For this review, take the finished solid that the model builds, in its own axes (mm). A direction names the side the tool comes from. Give positions to 0.01 mm unless a question says otherwise; leave off trailing zeros. Order: outer loops, then holes, each group sorted by start corner. A loop starts at its lowest first (then second) coordinate and runs counter-clockwise, first axis right, second up.
Item 1: For probe 1 along Y at (x, z) = (11.5, 2); probe 2 along Z at (x, y) = (48.5, 11); probe 3 along Y at (x, z) = (38.5, 4.5), list the stretches that pass through material, from the lowest coordinate up.
Item 2: Consider section C-C (y = -79). Give the boundary of the cut face in (x, z).
Item 3: Consider section B-B (x = 6). Give the boundary of the cut face in (y, z), plus the area to 3 significant figures.
Item 4: The part is to be moulded in two halves that separate along X. For faces 1 (the flat face through (-86.994, -51.168, 5.465)), 2 (the flat face through (-1, 1, 20)), 3 (the flat face through (-1, 102, 3)), 4 (the flat face through (-60.854, -102.443, -3.055)), say which applies: released by +X, released by -X, zero draft, split by the parting line, or undercut.
Item 5: Machinability: for faces 5 (the flat face through (60.854, 102.443, -3.055)), 6 (the flat face through (-0.79, -91.21, 13.47)), 7 (the flat face through (-1, 100.923, 5)), 8 (the flat face through (87.81, -49.755, 5.465)), which of the approach directions +Z, -Z, +X, -X, +Y, -Y give a long, thin tool a straight path to every point of the face, cutting with its end or side? Answer none if there is none.
Item 6: Consider section A-A (z = 15). Give the boundary of the cut face in (x, y).
Item 7: For P1, Ø1.5, axis at x = -19.5, z = 2, coming from the -Y side; P2, Ø3, axis at x = -25.5, z = 14, coming from the +Y side; P3, Ø2.5, axis at x = -120, y = -4.5, coming from the +Z side, all flat-tipped, find the tip position at first contact; note any pin that passes through.
Autodesk Inventor part; units mm, degrees
ref_plane "YZ Plane" through (0, 0, 0) normal (1, 0, 0) x (0, 1, 0)
ref_plane "XZ Plane" through (0, 0, 0) normal (0, 1, 0) x (-1, 0, 0)
ref_plane "XY Plane" through (0, 0, 0) normal (0, 0, 1) x (1, 0, 0)
ref_plane "Plano de trabajo1" through (0, 0, 0) normal (0, 0, 1) x (1, 0, 0)
sketch "Boceto1" plane through (0, 0, 0) normal (0, 0, 1) x (1, 0, 0)
  line L0 (58.8453, 101.923) -> (-58.8453, 101.923)
  line L1 (-58.8453, 101.923) -> (-117.6906, 0)
  line L2 (-117.6906, 0) -> (-58.8453, -101.923)
  line L3 (-58.8453, -101.923) -> (58.8453, -101.923)
  line L4 (58.8453, -101.923) -> (117.6906, 0)
  line L5 (117.6906, 0) -> (58.8453, 101.923)
  line L6 (-60, 103.923) -> (-120, 0)
  line L7 (-120, 0) -> (-60, -103.923)
  line L8 (-60, -103.923) -> (60, -103.923)
  line L9 (60, -103.923) -> (120, 0)
  line L10 (120, 0) -> (60, 103.923)
  line L11 (60, 103.923) -> (-60, 103.923)
  line L12 (58.8453, 101.923) -> (117.6906, 0)
  line L13 (117.6906, 0) -> (58.8453, -101.923)
  line L14 (58.8453, -101.923) -> (-58.8453, -101.923)
  line L15 (-58.8453, -101.923) -> (-117.6906, 0)
  line L16 (-117.6906, 0) -> (-58.8453, 101.923)
  line L17 (-58.8453, 101.923) -> (58.8453, 101.923)
  point P0 (0, 0)
extrude "Extrusión1" add sketch "Boceto1" along normal blind 3 contours L5 L4 L3 L2 L1 L0 | L11 L10 L9 L8 L7 L6
sketch "Boceto2" plane through (0, 0, 3) normal (0, 0, 1) x (1, 0, 0)
  line L0 (-120, 0) -> (-60, -103.923)
  line L1 (-60, -103.923) -> (60, -103.923)
  line L2 (60, -103.923) -> (120, 0)
  line L3 (120, 0) -> (60, 103.923)
  line L4 (60, 103.923) -> (-60, 103.923)
  line L5 (-60, 103.923) -> (-120, 0)
  line L6 (58.2679, 100.923) -> (116.5359, 0)
  line L7 (116.5359, 0) -> (58.2679, -100.923)
  line L8 (58.2679, -100.923) -> (-58.2679, -100.923)
  line L9 (-58.2679, -100.923) -> (-116.5359, 0)
  line L10 (-116.5359, 0) -> (-58.2679, 100.923)
  line L11 (-58.2679, 100.923) -> (58.2679, 100.923)
  point P0 (0, 0)
  dimension "d2" = 3
extrude "Extrusión2" add sketch "Boceto2" along normal blind 20 contours L6 L7 L8 L9 L10 L11
chamfer "Chaflán1" distance 15 angle 45 6 edges at (-87.4019, 50.4615, 23) (-87.4019, -50.4615, 23) (0, -100.923, 23) (87.4019, -50.4615, 23) (87.4019, 50.4615, 23) (0, 100.923, 23)
sketch "Boceto3" plane through (0, 0, 0) normal (0, 0, -1) x (-1, 0, 0)
  line L0 (117.6906, 0) -> (58.8453, -101.923)
  line L1 (58.8453, -101.923) -> (-58.8453, -101.923)
  line L2 (58.8453, 101.923) -> (117.6906, 0)
  line L3 (-117.6906, 0) -> (-58.8453, 101.923)
  line L4 (-58.8453, -101.923) -> (-117.6906, 0)
  point P0 (0, 0)
shell "Vaciado1" thickness 3 removed faces 1 at (-20, 34.641, 0)
sketch "Boceto4" plane through (-60, -103.923, 0) normal (-0.866, -0.5, 0) x (0, 0, 1)
  line L0 (0, 120) -> (0, 0)
  line L1 (0, 0) -> (3, 0)
  line L2 (3, 120) -> (3, 0)
  line L3 (0, 120) -> (3, 120)
  line L4 (0, 120) -> (3, 120)
  line L5 (0, 0) -> (0, 120)
  line L6 (3, 120) -> (0, 120)
  line L7 (0, 120) -> (0, 114)
  line L8 (0, 114) -> (3, 114)
  line L9 (3, 114) -> (3, 120)
  line L10 (0, 0) -> (3, 0)
  line L11 (3, 0) -> (3, 6)
  line L12 (3, 6) -> (0, 6)
  line L13 (0, 6) -> (0, 0)
  point P0 (0, 60)
  point P1 (0, 114)
  point P2 (3, 114)
  point P3 (0, 6)
  dimension "d9" = 6
  dimension "d10" = 6
extrude "Extrusión3" add sketch "Boceto4" along normal blind 3 contours L3 L2 L8 L0 | L12 L2 L1 L0
sketch "Boceto5" plane through (0, 0, 0) normal (0, 0, -1) x (-1, 0, 0)
  line L0 (-56.5359, 97.923) -> (56.5359, 97.923)
  line L1 (56.5359, 97.923) -> (113.0718, 0)
  line L2 (113.0718, 0) -> (56.5359, -97.923)
  line L3 (56.5359, -97.923) -> (-56.5359, -97.923)
  line L4 (-56.5359, -97.923) -> (-113.0718, 0)
  line L5 (-113.0718, 0) -> (-56.5359, 97.923)
  line L6 (60, 103.923) -> (120, 0)
  line L7 (-60, 103.923) -> (60, 103.923)
  line L8 (-120, 0) -> (-60, 103.923)
  line L9 (-60, -103.923) -> (-120, 0)
  line L10 (60, -103.923) -> (-60, -103.923)
  line L11 (60, -103.923) -> (62.5981, -105.423)
  line L12 (65.5981, -100.2269) -> (62.5981, -105.423)
  line L13 (63, -98.7269) -> (65.5981, -100.2269)
  line L14 (117, -5.1962) -> (63, -98.7269)
  line L15 (117, -5.1962) -> (119.5981, -6.6962)
  line L16 (122.5981, -1.5) -> (119.5981, -6.6962)
  line L17 (120, 0) -> (122.5981, -1.5)
  line L18 (120, 0) -> (117, -5.1962)
  line L19 (63, -98.7269) -> (60, -103.923)
  point P0 (0, 0)
extrude "Extrusión4" add sketch "Boceto5" along normal blind 8 contours L17 L16 L15 L18 | L13 L12 L11 L19
sketch "Boceto6" plane through (-62.5981, -105.423, 0) normal (-0.866, -0.5, 0) x (0, 0, 1)
  line L0 (3, 114) -> (-8, 114)
  line L1 (-8, 114) -> (-8, 117)
  line L2 (-8, 114) -> (-8, 120)
  line L3 (-8, 117) -> (-4.5, 117)
  circle A0 centre (-4.5, 117) radius 1.5
  line L4 (-8, 6) -> (-8, 0)
  line L5 (-8, 6) -> (-8, 3)
  line L6 (-8, 3) -> (-4.5, 3)
  circle A1 centre (-4.5, 3) radius 1.5
  point P0 (0, 60)
  dimension "d15" = 3.5
  dimension "d16" = 3
  dimension "d17" = 3.5
  dimension "d18" = 3
extrude "Extrusión5" cut sketch "Boceto6" against normal blind 8
sketch "Boceto7" plane through (60, 103.923, 3) normal (0.866, 0.5, 0) x (0, 0, -1)
  line L0 (3, -120) -> (3, 0)
  line L1 (3, 0) -> (0, 0)
  line L2 (0, -120) -> (0, 0)
  line L3 (3, -120) -> (0, -120)
  line L4 (3, -120) -> (0, -120)
  line L5 (0, -120) -> (0, -114)
  line L6 (0, -114) -> (3, -114)
  line L7 (3, -114) -> (3, -120)
  line L8 (3, 0) -> (0, 0)
  line L9 (0, 0) -> (0, -6)
  line L10 (0, -6) -> (3, -6)
  line L11 (3, -6) -> (3, 0)
  point P0 (3, -60)
  point P1 (3, -114)
  point P2 (3, -6)
  dimension "d21" = 6
  dimension "d22" = 6
extrude "Extrusión6" add sketch "Boceto7" along normal blind 3 contours L3 L2 L6 L0 | L10 L2 L1 L0
sketch "Boceto8" plane through (0, 0, 0) normal (0, 0, -1) x (-1, 0, 0)
  line L0 (-56.5359, 97.923) -> (56.5359, 97.923)
  line L1 (56.5359, 97.923) -> (113.0718, 0)
  line L2 (113.0718, 0) -> (56.5359, -97.923)
  line L3 (56.5359, -97.923) -> (-56.5359, -97.923)
  line L4 (-56.5359, -97.923) -> (-113.0718, 0)
  line L5 (-113.0718, 0) -> (-56.5359, 97.923)
  line L6 (60, -103.923) -> (63, -98.7269)
  line L7 (117, -5.1962) -> (63, -98.7269)
  line L8 (117, -5.1962) -> (120, 0)
  line L9 (60, 103.923) -> (120, 0)
  line L10 (-60, 103.923) -> (60, 103.923)
  line L11 (-60, 103.923) -> (-62.5981, 105.423)
  line L12 (-65.5981, 100.2269) -> (-62.5981, 105.423)
  line L13 (-63, 98.7269) -> (-65.5981, 100.2269)
  line L14 (-117, 5.1962) -> (-63, 98.7269)
  line L15 (-117, 5.1962) -> (-119.5981, 6.6962)
  line L16 (-122.5981, 1.5) -> (-119.5981, 6.6962)
  line L17 (-120, 0) -> (-122.5981, 1.5)
  line L18 (-60, -103.923) -> (-120, 0)
  line L19 (60, -103.923) -> (-60, -103.923)
  line L20 (-120, 0) -> (-60, 103.923)
  point P0 (0, 0)
  point P1 (-63, 98.7269)
  point P2 (-117, 5.1962)
extrude "Extrusión7" add sketch "Boceto8" along normal blind 8 contours L17 L16 L15 L20 | L13 L12 L11 L20
sketch "Boceto9" plane through (62.5981, 105.423, 3) normal (0.866, 0.5, 0) x (0, 0, -1)
  circle A0 centre (7.5, -117) radius 1.5
  circle A1 centre (7.5, -3) radius 1.5
  point P0 (3, -60)
extrude "Extrusión8" cut sketch "Boceto9" against normal blind 8
properties part number "tapaHEX"
Resolved:
1. probe 1: y = -103.92 to -97.92, 97.92 to 103.92
1. probe 2: z = 20 to 23
1. probe 3: y = -100.92 to -97.92, 97.92 to 100.92
2. outline: (-74.39, 0) - (-67.46, 0) - (-67.46, 6.76) - (-52.17, 20) - (52.17, 20) - (67.46, 6.76) - (67.46, 0) - (74.39, 0) - (74.39, 3) - (70.93, 3) - (70.93, 8) - (53.6, 23) - (-53.6, 23) - (-70.93, 8) - (-70.93, 3) - (-74.39, 3) - close
3. outline: (-103.92, 0) - (-97.92, 0) - (-97.92, 6.76) - (-84.68, 20) - (84.68, 20) - (97.92, 6.76) - (97.92, 0) - (103.92, 0) - (103.92, 3) - (100.92, 3) - (100.92, 8) - (85.92, 23) - (-85.92, 23) - (-100.92, 8) - (-100.92, 3) - (-103.92, 3) - close
3. area: 694 mm2
4. face 1: released by -X
4. face 2: undercut
4. face 3: zero draft
4. face 4: released by +X
5. face 5: -Z, -X, -Y
5. face 6: -Z
5. face 7: +Z, +X, -X, +Y
5. face 8: +Z, +X, -Y
6. outline: (-108.45, 0) - (-54.23, -93.92) - (54.23, -93.92) - (108.45, 0) - (54.23, 93.92) - (-54.23, 93.92) - close; hole (-103.55, 0) - (-51.78, -89.68) - (51.78, -89.68) - (103.55, 0) - (51.78, 89.68) - (-51.78, 89.68) - close
7. P1: stops at y = -103.92
7. P2: stops at y = 96.42
7. P3: stops at z = 3
